```python
from build123d import *

# Parameters (mm, degrees)
BOSS_EXTRUDE2_DEPTH = 762
FILLET2_R           = 1.27


with BuildPart() as part:
    # Sketch1 → Boss-Extrude2 (new body)
    with BuildSketch(Plane.XY):
        with BuildLine():
            Line((0, 0), (-4.7625, 0))
            Line((-4.7625, 0), (-4.7625, 5.55625))
            ThreePointArc((-4.7625, 5.55625), (-5.69243597, 7.80131403), (-7.9375, 8.73125))
            Line((-7.9375, 8.73125), (-7.9375, 28.575))
            Line((-7.9375, 28.575), (-11.1125, 28.575))
            ThreePointArc((-11.1125, 28.575), (-12.019610958, 38.289886849), (-16.522183488, 46.946024405))
            Line((-16.522183488, 46.946024405), (-20.049007231, 51.371088071))
            ThreePointArc((-20.049007231, 51.371088071), (-21.43125, 55.488518856), (-19.84375, 59.53125))
            Line((-19.84375, 59.53125), (-23.8125, 59.53125))
            Line((-23.8125, 59.53125), (-23.8125, 76.2))
            Line((-23.8125, 76.2), (0, 76.2))
            Line((0, 76.2), (0, 74.93))
            Line((0, 74.93), (-22.5425, 74.93))
            Line((-22.5425, 74.93), (-22.5425, 60.80125))
            Line((-22.5425, 60.80125), (-19.84375, 60.80125))
            ThreePointArc((-19.84375, 60.80125), (-18.686099129, 60.053499423), (-18.891651575, 58.690768834))
            ThreePointArc((-18.891651575, 58.690768834), (-20.161651575, 55.456583919), (-19.05585736, 52.162639291))
            Line((-19.05585736, 52.162639291), (-15.529033617, 47.737575625))
            ThreePointArc((-15.529033617, 47.737575625), (-11.00800601, 39.317919875), (-9.745436159, 29.845))
            Line((-9.745436159, 29.845), (-6.6675, 29.845))
            Line((-6.6675, 29.845), (-6.6675, 9.815959497))
            ThreePointArc((-6.6675, 9.815959497), (-4.373571339, 8.212645584), (-3.4925, 5.55625))
            Line((-3.4925, 5.55625), (-3.4925, 1.27))
            Line((-3.4925, 1.27), (0, 1.27))
            Line((0, 1.27), (0, 0))
        make_face()
    extrude(amount=-BOSS_EXTRUDE2_DEPTH)

    # Fillet2
    fillet2_edges = [part.edges().sort_by_distance(p)[0] for p in [
        (-6.6675, 29.845, -381),
        (-4.7625, 0, -381),
        (-7.9375, 8.73125, -381),
        (-11.1125, 28.575, -381),
        (-23.8125, 59.53125, -381),
        (-23.8125, 76.2, -381),
    ]]
    fillet(fillet2_edges, radius=FILLET2_R)


solid = part.part
```
Model file for the job. Use its own axes, mm. A direction names the side the tool comes from. Give positions to 0.01 mm unless a question says otherwise; leave off trailing zeros. Loops run counter-clockwise (first coordinate to the right, second up) from the corner with the lowest first, then second, coordinate; pieces in that order, holes last. Notation, with made-up numbers: (63, -36.5) - (106, -36.5) arc R14 cw to (106, -13.5) - close; hole circle Ø3 at (25.25, 82). An arc over 180 degrees is marked (long way). One line per item, written item: value. Start each with the question number.
1. Pull direction Y, two halves, no side cores. Call faces 1 (the flat face through (-11, 76.2, -376)), 2 (the flat face through (-7.938, 19, -376)), 3 (the flat face through (-11, 74.93, -376)): pulls with the +Y half, pulls with the -Y half, needs draft (parallel to the pull), parting line crosses it, or undercut.
2. Which spindle directions (+Z, -Z, +X, -X, +Y, -Y) get a long thin tool onto all of the face, cutting with end or side? Do faces 4 (the flat face through (-18, 50, 0)), 5 (the flat face through (-22.542, 68, -376)). Say none if no direction does.
3. Probe L1, parallel to Y at x = -22.25, z = -172; L2, parallel to Y at x = -19.25, z = -351.5; L3, parallel to X at y = 11, z = -302.5. List the from-to ranges inside material, lowest first. Write a range as from..to.
4. Slice it at A-A (y = 16.5). List the corners of the cut face in (x, z), plus the area to 3 significant figures.
5. Pin check, flat tips, straight feed: pin 1 (3 mm diameter, centred on x = -21, z = -558.5, fed in from -Y); pin 2 (1 mm diameter, centred on y = 46.5, z = -667, fed in from -X); pin 3 (1.3 mm diameter, centred on y = 3, z = -351.5, fed in from -X). Stop position of each tip, or through.
Solution:
1. face 1: pulls with the +Y half
1. face 2: needs draft
1. face 3: undercut
2. face 4: +Z, +X, -X, +Y, -Y
2. face 5: +Z, -Z, +X
3. L1: y = 59.53..60.8, 74.93..76.2
3. L2: y = 50.37..52.42, 58.23..60.65, 74.93..76.2
3. L3: x = -7.94..-6.67
4. outline: (-7.94, -762) - (-6.67, -762) - (-6.67, 0) - (-7.94, 0) - close
4. area: 968 mm^2
5. pin 1: stops at y = 50.68
5. pin 2: stops at x = -16.57
5. pin 3: stops at x = -4.76
